The model under review builds one solid part; all positions refer to its coordinate system, in mm. Face numbers are marked on the shaded views. Give positions to 0.01 mm unless a question says otherwise; leave off trailing zeros. Use CSV: the item, a comma, the result in double quotes.
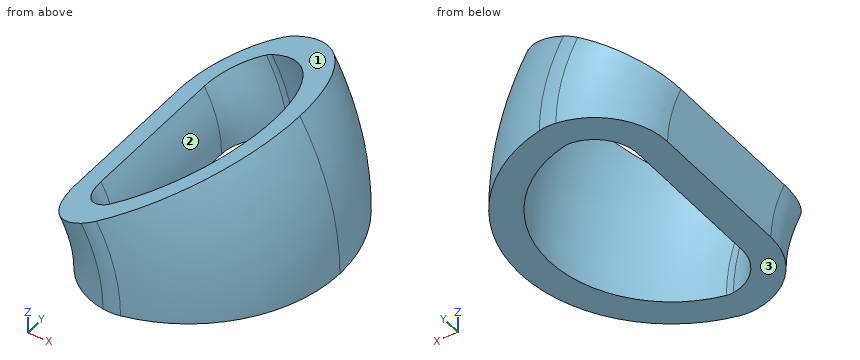
Autodesk Inventor part; units mm, degrees
ref_plane "Work Plane2" through (0, 0, 0) normal (-0.2588, 0, -0.9659) x (0, 1, 0)
ref_plane "Work Plane1" through (-7, 0, -29.5697) normal (1, 0, 0) x (0, 0, -1)
ref_plane "YZ Plane" through (0, 0, 0) normal (1, 0, 0) x (0, 1, 0)
sketch "Sketch1" plane through (0, 0, 0) normal (0, 0, 1) x (1, 0, 0)
  line L0 (0, 0) -> (0, 15.36) construction
  line L1 (10.24, 7.86) -> (10.24, -7.86)
  line L2 (17.74, 15.36) -> (17.74, -15.36) construction
  arc A0 (16.6996, 15.2875) -> (10.24, 7.86) centre (17.74, 7.86) ccw
  arc A1 (10.24, -7.86) -> (16.6996, -15.2875) centre (17.74, -7.86) ccw
  arc A2 (18.4574, -15.2213) -> (18.4574, 15.2213) centre (15.1418, 0) ccw
  line L3 (0, 0) -> (51.4073, 0)
  arc A3 (18.4574, 15.2213) -> (16.6996, 15.2875) centre (17.3932, 10.3358) ccw
  arc A4 (16.6996, -15.2875) -> (18.4574, -15.2213) centre (17.3932, -10.3358) ccw
  arc A5 (17.8189, 12.29) -> (17.1158, 12.3165) centre (17.3932, 10.3358) ccw
  arc A6 (17.1158, 12.3165) -> (13.24, 7.86) centre (17.74, 7.86) ccw
  line L4 (13.24, 7.86) -> (13.24, -7.86)
  arc A7 (13.24, -7.86) -> (17.1158, -12.3165) centre (17.74, -7.86) ccw
  arc A8 (17.1158, -12.3165) -> (17.8189, -12.29) centre (17.3932, -10.3358) ccw
  arc A9 (17.8189, -12.29) -> (17.8189, 12.29) centre (15.1418, 0) ccw
  point P0 (10.24, 0)
  point P1 (30.72, 0)
  point P2 (17.74, 0)
  dimension "MaxHeight" = 15.36
  dimension "FlatHeightx2" = 15.72
  dimension "ID" = 20.48
  dimension "OD" = 61.44
  dimension "d5" = 30.72
  dimension "RadAtPeak" = 17.74
  dimension "d90" = 5
  dimension "d97" = 3
revolve "Revolution1" add sketch "Sketch1" angle 30 about axis through (0, 0, 0) along (0, -1, 0) contours A0 A3 A2 L3 A9 A5 A6 L4 L1 | L3 L4 A7 A8 A9 A2 A4 A1 L1
sketch "Sketch7" plane through (0, 0, 0) normal (0, 1, 0) x (-1, 0, 0)
  circle A0 centre (0, 0) radius 198.9616
sketch "Sketch8" plane through (0, 0, 0) normal (1, 0, 0) x (0, 1, 0)
  circle A0 centre (0, 0) radius 159.0195
sketch "Sketch9" plane through (0, 0, 0) normal (1, 0, 0) x (0, 0, -1)
  line L0 (74, 0) -> (35, 0)
  point P0 (0, 0)
  point P1 (-52.5, 0)
  point P2 (0, 0)
  point P3 (52.5, 0)
  dimension "d88" = 105
  dimension "d89" = 52.5
sketch "Sketch11" plane through (0, 0, 0) normal (1, 0, 0) x (0, 0, -1)
  arc A0 (-35, 25.9107) -> (-42.6927, 34.8921) centre (-44.0893, 25.9107) ccw
  line L0 (-35, 25.9107) -> (-35, 0)
  line L1 (-35, 0) -> (35, 0)
  arc A1 (-50.0415, 0) -> (-54.9585, 0) centre (-52.5, 0) ccw
  arc A2 (-50.0415, 0) -> (-54.9585, 0) centre (-37.5, 0) ccw
  arc A3 (-39.8678, 39.0634) -> (-73, 0) centre (-33.4058, 0) ccw
  arc A4 (-29.5697, 27.789) -> (-36.4391, 38.3935) centre (-44.0893, 25.9107) ccw
  line L2 (-29.5697, 27.789) -> (-29.5697, 0)
  line L3 (-35, 0) -> (35, 0)
  line L4 (-73, 0) -> (-29.5697, 0)
  arc A5 (-36.4391, 38.3935) -> (-39.8678, 39.0634) centre (-39.0518, 34.1304) ccw
  point P0 (0, 0)
  point P1 (-35, 0)
  point P2 (-29.5697, 0)
  point P3 (-54.9585, 0)
  point P4 (-50.0415, 0)
  dimension "d91" = 5
equation "\"d5\" = 2 * MaxHeight"
equation "\"d63_Copy\" = 35"
properties part number "L_20uH-Wedge" material "UHMW, White"
Q1. To check wall thickness, follow probe 1 along X at (y, z) = (1, 5.5); probe 2 along X at (y, z) = (11, 1.75); probe 3 along Y at (x, z) = (23.75, 5.75). State the ranges of each line that lie inside material, in increasing order.
Derived:
probe 1,"x = 9.53 to 12.04, 27.13 to 30.19"
probe 2,"x = 10.79 to 14.41, 21.17 to 26.11"
probe 3,"y = -12.5 to -8.48, 8.48 to 12.5"
Q2. Insertion check: pin 1 (5 mm diameter, centred on y = 0.5, z = 12.5, fed in from +X); pin 2 (1 mm diameter, centred on y = -10, z = 13.5, fed in from +X); pin 3 (2 mm diameter, centred on x = 21.5, z = 9.5, fed in from +Y); pin 4 (5 mm diameter, centred on x = 24.5, y = 6.5, fed in from -Z). Each pin has a flat end and moves straight along its axis. Give the tip position at first contact, or say it passes through.
Derived:
pin 1,"stops at x = 29.04"
pin 2,"stops at x = 24.02"
pin 3,"stops at y = 13.73"
pin 4,"stops at z = 0"
Q3. The part is to be moulded in two halves that separate along X. For the marked faces 1, 2 and 3, say which applies: pulls with the +X half, pulls with the -X half, needs draft (parallel to the pull), parting line crosses it, or undercut.
Derived:
face 1,"pulls with the -X half"
face 2,"undercut"
face 3,"needs draft"
